The model under review builds one solid part; all positions refer to its coordinate system, in mm. Coordinates: 2 decimals unless noted, no trailing zeros. Order: outer loops, then holes, each group sorted by start corner. A loop starts at its lowest first (then second) coordinate and runs counter-clockwise, first axis right, second up. Notation, with made-up numbers: (64.5, 49) -> (73.5, 49) arc R13 ccw to (73.5, 62) -> close; hole circle Ø11 at (3, 85). An arc over 180 degrees is marked (long way). Answer as CSV lines item,"result". Start each with the question number.
from build123d import *

# Parameters (mm, degrees)
SKETCH_1_R          = 10
EXTRUDE_1_DEPTH     = 520
SKETCH_2_R          = 4.3
CUT_EXTRUDE_2_DEPTH = 25
CHAMFER_1_SIZE      = 1


with BuildPart() as part:
    # 草图1 → 拉伸1 (new body)
    with BuildSketch(Plane(origin=(0, 0, 0), x_dir=(0, 0, -1), z_dir=(1, 0, 0))):
        Circle(SKETCH_1_R)
    extrude(amount=EXTRUDE_1_DEPTH)

    # 草图2 → 拉伸2 (cut)
    with BuildSketch(Plane(origin=(520, 0, 0), x_dir=(0, 0, -1), z_dir=(1, 0, 0))):
        Circle(SKETCH_2_R)
    extrude(amount=-CUT_EXTRUDE_2_DEPTH, mode=Mode.SUBTRACT)

    # 倒角1
    chamfer_1_edges = [part.edges().sort_by_distance(p)[0] for p in [
        (520, 0, 4.3),
    ]]
    chamfer(chamfer_1_edges, length=CHAMFER_1_SIZE)


solid = part.part
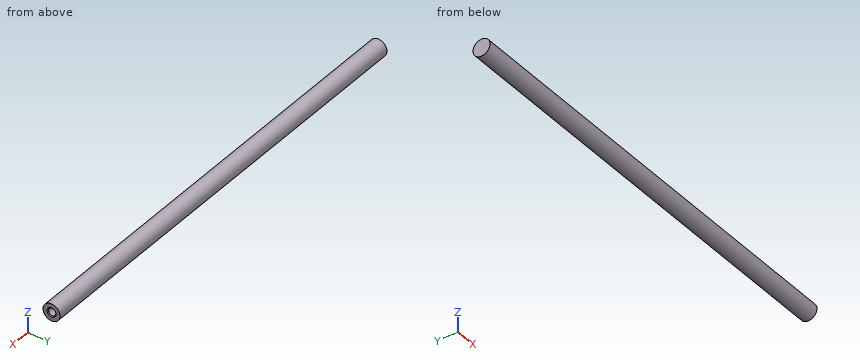
1) Insertion check: pin 1 Ø12 at (x, y) = (201, 2.5) entering from -Z; pin 2 Ø10 at (x, z) = (433.5, 7) entering from +Y; pin 3 Ø2.5 at (y, z) = (1, 1.5) entering from +X. Each pin has a flat end and moves straight along its axis. Give the tip position at first contact, or say it passes through.
2) Wall thickness on L1, parallel to Y at x = 505, z = 0; L2, parallel to Y at x = 238, z = 8.5; L3, parallel to X at y = 4, z = -0.5: over which ranges is each line inside the solid? List them lowest first. Write a range as [from, to].
3) Consider section C-C (x = 98.5). Give the boundary of the cut face in (y, z), plus the area to 3 significant figures.
4) Consider section A-A (z = 0). Give the boundary of the cut face in (x, y).
Result:
1,pin 1,"z = -10"
1,pin 2,"y = 9.8"
1,pin 3,"x = 495"
2,L1,"[-10, -4.3], [4.3, 10]"
2,L2,"[-5.27, 5.27]"
2,L3,"[0, 495]"
3,outline,"circle Ø20 at (0, 0)"
3,area,"314 mm2"
4,outline,"(0, -10) -> (520, -10) -> (520, -5.3) -> (519, -4.3) -> (495, -4.3) -> (495, 4.3) -> (519, 4.3) -> (520, 5.3) -> (520, 10) -> (0, 10) -> close"
